Model file for the job. Use its own axes, mm. Face numbers are marked on the shaded views. A direction names the side the tool comes from. Round coordinates to 2 decimals unless told otherwise and drop trailing zeros. Order: outer loops, then holes, each group sorted by start corner. A loop starts at its lowest first (then second) coordinate and runs counter-clockwise, first axis right, second up. Notation, with made-up numbers: (-2, 73.5) - (16, 73.5) arc R17 ccw to (16, 92.5) - close; hole circle Ø9 at (7.25, -24.5). An arc over 180 degrees is marked (long way). Write item = value, one per line.
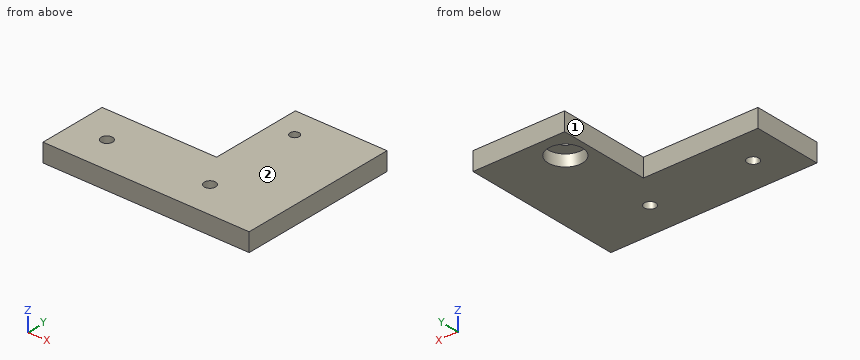
```python
from build123d import *

# Parameters (mm, degrees)
SKETCH1_R           = 2.5
BOSS_EXTRUDE1_DEPTH = 8
SKETCH2_R           = 7.5
CUT_EXTRUDE1_DEPTH  = 5
SKETCH3_R           = 2
CUT_EXTRUDE2_DEPTH  = 114.791165634


with BuildPart() as part:
    # Sketch1 → Boss-Extrude1 (new body)
    with BuildSketch(Plane.XY):
        Polygon((-50.724939449, 17.294061535), (-10.724939449, 17.294061535), (-10.724939449, -52.705938465), (-100.724939449, -52.705938465), (-100.724939449, -22.705938465), (-50.724939449, -22.705938465), align=None)
        with Locations((-85.724939449, -37.705938465)):
            Circle(SKETCH1_R, mode=Mode.SUBTRACT)
        with Locations((-40.724939449, -37.705938465)):
            Circle(SKETCH1_R, mode=Mode.SUBTRACT)
    extrude(amount=BOSS_EXTRUDE1_DEPTH)

    # Sketch2 → Cut-Extrude1 (cut)
    with BuildSketch(Plane(origin=(0, 0, 0), x_dir=(-1, 0, 0), z_dir=(0, 0, -1))):
        with Locations((40.724939449, 5.294061535)):
            Circle(SKETCH2_R)
    extrude(amount=-CUT_EXTRUDE1_DEPTH, mode=Mode.SUBTRACT)

    # Sketch3 → Cut-Extrude2 (cut, through all)
    with BuildSketch(Plane(origin=(0, 0, 5), x_dir=(-1, 0, 0), z_dir=(0, 0, -1))):
        with Locations((40.724939449, 5.294061535)):
            Circle(SKETCH3_R)
    extrude(amount=-CUT_EXTRUDE2_DEPTH, mode=Mode.SUBTRACT)


solid = part.part
```
1) Wall check: line 1 along X through (y, z) = (-40, 2.25); line 2 along X through (y, z) = (-13.5, 3); line 3 along Y through (x, z) = (-94.5, 1.5). Give the ranges that are in metal, low to high.
Conclusion:
line_1 = -100.72 to -86.72, -84.73 to -41.72, -39.73 to -10.72
line_2 = -50.72 to -10.72
line_3 = -52.71 to -22.71
2) 3-axis set-ups, long thin cutter, end or side, ignore diameter. For the marked faces 1 and 2: which of +Z, -Z, +X, -X, +Y, -Y reach the whole face in a straight line?
Conclusion:
face_1 = +Z, -Z, -X, +Y
face_2 = +Z, +X, -X, +Y, -Y
3) Cut at B-B (x = -34.5). Write the cut outline in (y, z), and give its area (3 significant figures).
Conclusion:
outline = (-52.71, 0) - (1.11, 0) - (1.11, 5) - (9.48, 5) - (9.48, 0) - (17.29, 0) - (17.29, 8) - (-52.71, 8) - close
area = 518 mm^2
4) Cut at A-A (z = 2.25). Write the cut outline in (x, y).
Conclusion:
outline = (-100.72, -52.71) - (-10.72, -52.71) - (-10.72, 17.29) - (-50.72, 17.29) - (-50.72, -22.71) - (-100.72, -22.71) - close; hole circle Ø5 at (-85.72, -37.71); hole circle Ø15 at (-40.72, 5.29); hole circle Ø5 at (-40.72, -37.71)
5) Cut at D-D (x = -79). Write the cut outline in (y, z), and give its area (3 significant figures).
Conclusion:
outline = (-52.71, 0) - (-22.71, 0) - (-22.71, 8) - (-52.71, 8) - close
area = 240 mm^2
6) Cut at C-C (z = 7). Write the cut outline in (x, y).
Conclusion:
outline = (-100.72, -52.71) - (-10.72, -52.71) - (-10.72, 17.29) - (-50.72, 17.29) - (-50.72, -22.71) - (-100.72, -22.71) - close; hole circle Ø5 at (-85.72, -37.71); hole circle Ø5 at (-40.72, -37.71); hole circle Ø4 at (-40.72, 5.29)
7) Flat gauge pins, fed straight in: pin 1 Ø4 at (y, z) = (-5, 3.5) entering from -X; pin 2 Ø3 at (x, y) = (-40.72, 5.29) entering from +Z; pin 3 Ø4.5 at (x, y) = (-37.5, 5) entering from -Z. Where does each tip first touch, or does it go through?
Conclusion:
pin_1 = -50.72
pin_2 = through
pin_3 = 5
